The listing builds one solid part. Answer for the finished solid, in the listing's coordinates (mm). Give positions to 0.01 mm unless a question says otherwise; leave off trailing zeros. Loops run counter-clockwise (first coordinate to the right, second up) from the corner with the lowest first, then second, coordinate; pieces in that order, holes last. Notation, with made-up numbers: M 81,48.25 L 138,48.25 A10 cw 138,54.25 Z; hole C -33.5,61 d9. An arc over 180 degrees is marked long. One line per item, written item: value. Start each with the question number.
Q1. A cutting plane is placed at B-B, the plane y = 3.5. Determine the outline of the cut face in (x, z).
Q2. A cutting plane is placed at A-A, the plane z = 7. Determine the outline of the cut face in (x, y).
Q3. Consider L1, parallel to X at y = 1.5, z = 90; L2, parallel to X at y = 4.75, z = 22; L3, parallel to Z at x = -90, y = 4.5. Determine where each line is inside the solid, lowest interval first.
Q4. A cutting plane is placed at C-C, the plane x = 96. Determine the outline of the cut face in (y, z), and give its area (3 significant figures).
Q5. A flat-ended cylindrical pin translates along its axis: pin 1 (3 mm diameter, centred on x = 90, z = 90, fed in from -Y). Find the tip coordinate at first contact, or state that the pin passes through.
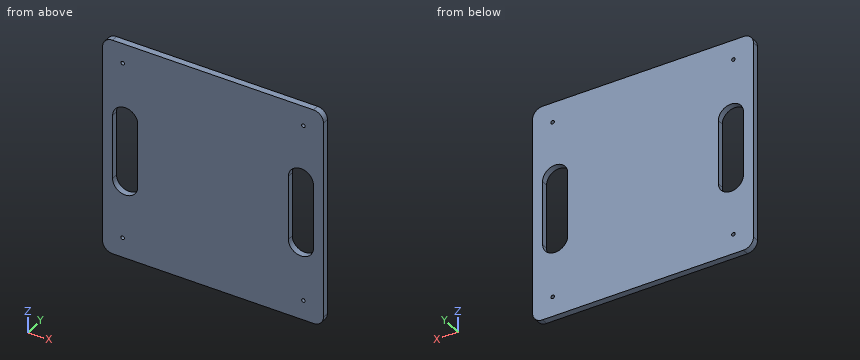
from build123d import *

# Parameters (mm, degrees)
SKETCH2_W           = 220
SKETCH2_H           = 220
BOSS_EXTRUDE1_DEPTH = 6.35
SKETCH3_R           = 1.8
CUT_EXTRUDE1_DEPTH  = 6.35
FILLET1_R           = 10
CUT_EXTRUDE2_DEPTH  = 10


with BuildPart() as part:
    # Sketch2 → Boss-Extrude1 (new body)
    with BuildSketch(Plane(origin=(0, 0, 0), x_dir=(1, 0, 0), z_dir=(0, 1, 0))):
        Rectangle(SKETCH2_W, SKETCH2_H)
    extrude(amount=BOSS_EXTRUDE1_DEPTH)

    # Sketch3 → Cut-Extrude1 (cut)
    with BuildSketch(Plane(origin=(0, 0, 0), x_dir=(-1, 0, 0), z_dir=(0, -1, 0))):
        with Locations((90, -90)):
            Circle(SKETCH3_R)
        with Locations((90, 90)):
            Circle(SKETCH3_R)
        with Locations((-90, 90)):
            Circle(SKETCH3_R)
        with Locations((-90, -90)):
            Circle(SKETCH3_R)
    extrude(amount=-CUT_EXTRUDE1_DEPTH, mode=Mode.SUBTRACT)

    # Fillet1
    fillet1_edges = [part.edges().sort_by_distance(p)[0] for p in [
        (110, 3.175, 110),
        (-110, 3.175, 110),
        (-110, 3.175, -110),
        (110, 3.175, -110),
    ]]
    fillet(fillet1_edges, radius=FILLET1_R)

    # Sketch7 → Cut-Extrude2 (cut)
    with BuildSketch(Plane(origin=(0, 6.35, 0), x_dir=(1, 0, 0), z_dir=(0, 1, 0))):
        with BuildLine():
            Line((-100, 32.5), (-100, -32.5))
            ThreePointArc((-100, -32.5), (-87.5, -45), (-75, -32.5))
            Line((-75, -32.5), (-75, 32.5))
            ThreePointArc((-75, 32.5), (-87.5, 45), (-100, 32.5))
        make_face()
        with BuildLine():
            Line((75, 32.5), (75, -32.5))
            ThreePointArc((75, -32.5), (87.5, -45), (100, -32.5))
            Line((100, -32.5), (100, 32.5))
            ThreePointArc((100, 32.5), (87.5, 45), (75, 32.5))
        make_face()
    extrude(amount=-CUT_EXTRUDE2_DEPTH, mode=Mode.SUBTRACT)


solid = part.part
Answer block:
1. outline: M -110,-100 A10 ccw -100,-110 L 100,-110 A10 ccw 110,-100 L 110,100 A10 ccw 100,110 L -100,110 A10 ccw -110,100 Z; hole M -100,-32.5 A12.5 ccw -75,-32.5 L -75,32.5 A12.5 ccw -100,32.5 Z; hole C -90,-90 d3.6; hole C -90,90 d3.6; hole M 75,-32.5 A12.5 ccw 100,-32.5 L 100,32.5 A12.5 ccw 75,32.5 Z; hole C 90,-90 d3.6; hole C 90,90 d3.6
2. outline: M -110,0 L -100,0 L -100,6.35 L -110,6.35 Z; M -75,0 L 75,0 L 75,6.35 L -75,6.35 Z; M 100,0 L 110,0 L 110,6.35 L 100,6.35 Z
3. L1: -110 to -91.8, -88.2 to 88.2, 91.8 to 110
3. L2: -110 to -100, -75 to 75, 100 to 110
3. L3: -110 to -91.8, -88.2 to -44.75, 44.75 to 88.2, 91.8 to 110
4. outline: M 0,-110 L 6.35,-110 L 6.35,-41.67 L 0,-41.67 Z; M 0,41.67 L 6.35,41.67 L 6.35,110 L 0,110 Z
4. area: 868 mm^2
5. pin 1: through
